The drawing under review shows one solid part. Ordinate dimensions are in mm from its lowest x, y, z. Give positions to 0.01 mm unless a question says otherwise; leave off trailing zeros. Loops run counter-clockwise (first coordinate to the right, second up) from the corner with the lowest first, then second, coordinate; pieces in that order, holes last. Notation, with made-up numbers: M 89,0 L 119,0 A18 cw 119,31 Z; hole C 77,-33.5 d11. An arc over 180 degrees is marked long. Answer as CSV lines item,"result".
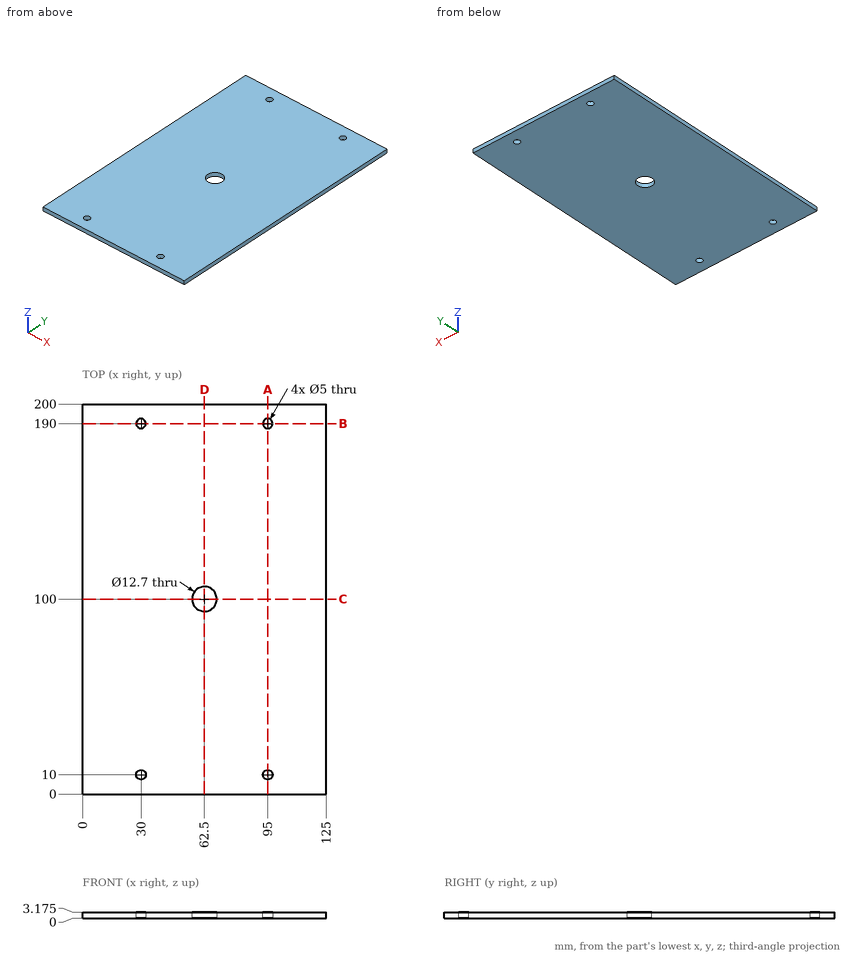
1. We need section B-B, the plane y = 190. Write out the cut boundary in (x, z) (3 decimals), plus the area to 3 significant figures.
Answer block:
outline,"M 0,0 L 27.5,0 L 27.5,3.175 L 0,3.175 Z; M 32.5,0 L 92.5,0 L 92.5,3.175 L 32.5,3.175 Z; M 97.5,0 L 125,0 L 125,3.175 L 97.5,3.175 Z"
area,"365 mm²"
2. We need section A-A, the plane x = 95. Write out the cut boundary in (y, z) (3 decimals), plus the area to 3 significant figures.
Answer block:
outline,"M 0,0 L 7.5,0 L 7.5,3.175 L 0,3.175 Z; M 12.5,0 L 187.5,0 L 187.5,3.175 L 12.5,3.175 Z; M 192.5,0 L 200,0 L 200,3.175 L 192.5,3.175 Z"
area,"603 mm²"
3. For P1, Ø3, axis at x = 95, y = 190, coming from the +Z side, flat-tipped, find the tip position at first contact; note if it passes through.
Answer block:
P1,"through"
4. We need section C-C, the plane y = 100. Write out the cut boundary in (x, z) (3 decimals).
Answer block:
outline,"M 0,0 L 56.15,0 L 56.15,3.175 L 0,3.175 Z; M 68.85,0 L 125,0 L 125,3.175 L 68.85,3.175 Z"
5. To check wall thickness, follow L1, parallel to X at y = 10, z = 1.25; L2, parallel to Y at x = 30, z = 1.65; L3, parallel to Y at x = 62.5, z = 1.4. State the ranges of each line that lie inside material, in increasing order. Write a range as [from, to].
Answer block:
L1,"[0, 27.5], [32.5, 92.5], [97.5, 125]"
L2,"[0, 7.5], [12.5, 187.5], [192.5, 200]"
L3,"[0, 93.65], [106.35, 200]"
6. We need section D-D, the plane x = 62.5. Write out the cut boundary in (y, z) (3 decimals), plus the area to 3 significant figures.
Answer block:
outline,"M 0,0 L 93.65,0 L 93.65,3.175 L 0,3.175 Z; M 106.35,0 L 200,0 L 200,3.175 L 106.35,3.175 Z"
area,"595 mm²"
